Geometry: final body of the model. Coordinates: model frame, mm. A direction names the side the tool comes from. Give positions to 0.01 mm unless a question says otherwise; leave off trailing zeros. Loops run counter-clockwise (first coordinate to the right, second up) from the corner with the lowest first, then second, coordinate; pieces in that order, holes last.
from build123d import *

# Parameters (mm, degrees)
F1_DEPTH = 40
F2_SIZE2 = 7.0020753821
F2_SIZE  = 10
F3_R     = 0.6
F4_R     = 3


with BuildPart() as f1:
    # F0 (on Top) → F1 (new body)
    with BuildSketch(Plane.XY):
        Polygon((9.6920941323, -33.465231495), (9.6920941323, 5.034768505), (32.6920941323, 5.034768505), (32.6920941323, -9.965231495), (34.1920941323, -9.965231495), (34.1920941323, 6.534768505), (8.1920941323, 6.534768505), (8.1920941323, -31.965231495), (-6.8079058677, -31.965231495), (-6.8079058677, -18.465231495), (-8.3079058677, -18.465231495), (-8.3079058677, -33.465231495), align=None)
    extrude(amount=F1_DEPTH)

    # F2
    f2_edges = [f1.edges().sort_by_distance(p)[0] for p in [
        (-7.557906, -18.465231, 40),
        (-7.557906, -18.465231, 0),
    ]]
    f2_side = f1.faces().sort_by_distance((-7.557906, -18.465231, 20))[0]
    chamfer(f2_edges, length=F2_SIZE, length2=F2_SIZE2, reference=f2_side)

    # F3
    f3_edges = [f1.edges().sort_by_distance(p)[0] for p in [
        (8.192094, 6.534769, 20),
        (9.692094, 5.034769, 20),
        (34.192094, -9.965231, 20),
        (32.692094, -9.965231, 20),
        (32.692094, 5.034769, 20),
        (34.192094, 6.534769, 20),
        (-6.807906, -18.465231, 20),
        (9.692094, -33.465231, 20),
        (-8.307906, -18.465231, 20),
        (-8.307906, -33.465231, 20),
        (-6.807906, -21.966269, 5),
        (-7.557906, -18.465231, 10),
        (-7.557906, -25.467307, 0),
        (-8.307906, -21.966269, 5),
        (-6.807906, -21.966269, 35),
        (-7.557906, -18.465231, 30),
        (-7.557906, -25.467307, 40),
        (-8.307906, -21.966269, 35),
    ]]
    fillet(f3_edges, radius=F3_R)

    # F4
    f4_edges = [f1.edges().sort_by_distance(p)[0] for p in [
        (8.192094, -31.965231, 20),
        (-6.807906, -31.965231, 20),
    ]]
    fillet(f4_edges, radius=F4_R)


solid = f1.part
Item 1: Ray query, probe 1 along X at (y, z) = (4.5, 18.5); probe 2 along X at (y, z) = (-26.5, 17); probe 3 along X at (y, z) = (-15, 38). Return the intervals inside material, ascending.
Values follow:
probe 1: x = 8.19 to 9.7, 32.69 to 34.19
probe 2: x = -8.31 to -6.81, 8.19 to 9.69
probe 3: x = 8.19 to 9.69
Item 2: Set-up query: faces 1 (the face through (-7, -22.3, 4.8)), 2 (the face through (9.692, -14, 20)), 3 (the face through (7.3, -31.1, 20.3)). Return all of +Z, -Z, +X, -X, +Y, -Y with unobstructed straight access to the full face (end or side cutting, diameter ignored); none if empty.
Values follow:
face 1: -Z, +Y
face 2: +Z, -Z, -Y
face 3: +Z, -Z, +Y
Item 3: Pin query (flat end, axial travel): pin 1 (6 mm diameter, centred on x = 12.5, z = 20, fed in from -Y); pin 2 (6.5 mm diameter, centred on x = 20, z = 18, fed in from -Y); pin 3 (6 mm diameter, centred on x = -2, z = 7, fed in from +Y). Return the tip coordinate at first contact, or that it passes through.
Values follow:
pin 1: stops at y = -33.31
pin 2: stops at y = 5.03
pin 3: stops at y = -31.72
Item 4: Section query B-B on z = 26. Return loops of the section in (x, y), plus the area to 3 significant figures.
Values follow:
outline: (-8.31, -32.87) arc R0.6 ccw to (-7.71, -33.47) - (9.09, -33.47) arc R0.6 ccw to (9.69, -32.87) - (9.69, 4.43) arc R0.6 cw to (10.29, 5.03) - (32.09, 5.03) arc R0.6 cw to (32.69, 4.43) - (32.69, -9.37) arc R0.6 ccw to (33.29, -9.97) - (33.59, -9.97) arc R0.6 ccw to (34.19, -9.37) - (34.19, 5.93) arc R0.6 ccw to (33.59, 6.53) - (8.79, 6.53) arc R0.6 ccw to (8.19, 5.93) - (8.19, -28.97) arc R3 cw to (5.19, -31.97) - (-3.81, -31.97) arc R3 cw to (-6.81, -28.97) - (-6.81, -19.07) arc R0.6 ccw to (-7.41, -18.47) - (-7.71, -18.47) arc R0.6 ccw to (-8.31, -19.07) - close
area: 168 mm2
Item 5: Section query A-A on y = -0.5. Return loops of the section in (x, z), plus the area to 3 significant figures.
Values follow:
outline: (8.19, 0) - (9.69, 0) - (9.69, 40) - (8.19, 40) - close; (32.69, 0) - (34.19, 0) - (34.19, 40) - (32.69, 40) - close
area: 120 mm2
Item 6: Section query D-D on y = -17.5. Return loops of the section in (x, z).
Values follow:
outline: (8.19, 0) - (9.69, 0) - (9.69, 40) - (8.19, 40) - close
Item 7: Section query C-C on x = 0.5. Return loops of the section in (y, z), plus the area to 3 significant figures.
Values follow:
outline: (-33.47, 0) - (-31.97, 0) - (-31.97, 40) - (-33.47, 40) - close
area: 60.0 mm2
